Autodesk Inventor part; units mm, degrees
ref_plane "YZ Plane" through (0, 0, 0) normal (1, 0, 0) x (0, 1, 0)
ref_plane "XZ Plane" through (0, 0, 0) normal (0, 1, 0) x (-1, 0, 0)
ref_plane "XY Plane" through (0, 0, 0) normal (0, 0, 1) x (1, 0, 0)
sketch "Szkic1" plane through (0, 0, 0) normal (0, 1, 0) x (-1, 0, 0)
  line L0 (0, 3.2611) -> (1.85, 3.2611)
  line L1 (1.85, 3.2611) -> (2.85, 2.6611)
  line L2 (2.85, 2.6611) -> (2.85, -6.3389)
  line L3 (2.85, -6.3389) -> (6.25, -6.3389)
  line L4 (6.25, -6.3389) -> (6.25, -7.9389)
  line L5 (6.25, -7.9389) -> (3.05, -7.9389)
  line L6 (3.05, -7.9389) -> (3.05, -33.9389)
  line L7 (3.05, -33.9389) -> (2.38, -35.4389)
  line L8 (2.38, -35.4389) -> (2.38, -36.3889)
  line L9 (2.38, -36.3889) -> (0, -38.5259)
  line L10 (0, 3.2611) -> (0, -38.5259)
  point P0 (0, 0)
  dimension "d0" = 1.85
  dimension "d1" = 0.6
  dimension "d2" = 1
  dimension "d3" = 9
  dimension "d4" = 3.4
  dimension "d5" = 1.6
  dimension "d6" = 3.2
  dimension "d7" = 26
  dimension "d8" = 1.5
  dimension "d9" = 0.67
  dimension "d10" = 0.95
  dimension "d11" = 2.137
revolve "Obrót1" add sketch "Szkic1" angle 360 about axis through (0, 0, 3.2611) along (0, 0, -1)
sketch "Szkic2" plane through (0, 0, -6.3389) normal (0, 0, 1) x (1, 0, 0)
  circle A0 centre (0, 0) radius 1.85
  line L0 (5.0074, 2.8738) -> (4.9925, -2.8997)
  line L1 (4.9925, -2.8997) -> (-0.0149, -5.7735)
  line L2 (-0.0149, -5.7735) -> (-5.0074, -2.8738)
  line L3 (-5.0074, -2.8738) -> (-4.9925, 2.8997)
  line L4 (-4.9925, 2.8997) -> (0.0149, 5.7735)
  line L5 (0.0149, 5.7735) -> (5.0074, 2.8738)
  circle A1 centre (0, 0) radius 5
  point P0 (0, 0)
  dimension "d13" = 10
sketch "Szkic3" plane through (0, 0, -7.9389) normal (0, 0, -1) x (-1, 0, 0)
  point P0 (0, 0)
extrude "Wyciągnięcie proste1" add sketch "Szkic2" along normal blind 5.2 contours A0 | L0 L1 A1 | L0 A1 L5 | A1 | A1 L4 L5 | L1 L2 A1 | A1 L3 L4 | L2 L3 A1
thread "Gwint1"
sketch "Szkic4" plane through (0, 0, -7.9389) normal (0, 0, -1) x (-1, 0, 0)
  point P0 (0, 0)
sketch "Szkic5" plane through (5.0074, 2.8738, -1.1389) normal (1, -0.0026, 0) x (0, 0, -1)
  point P0 (-1.1389, -2.8868)
sketch "Szkic6" plane through (0, 0, -7.9389) normal (0, 0, -1) x (-1, 0, 0)
  point P0 (0, 0)
sketch "Szkic7" plane through (5.0074, 2.8738, -1.1389) normal (1, -0.0026, 0) x (0, 0, -1)
  point P0 (-1.1389, -2.8868)
properties part number "śróbki1" material "Stal nierdzewna"
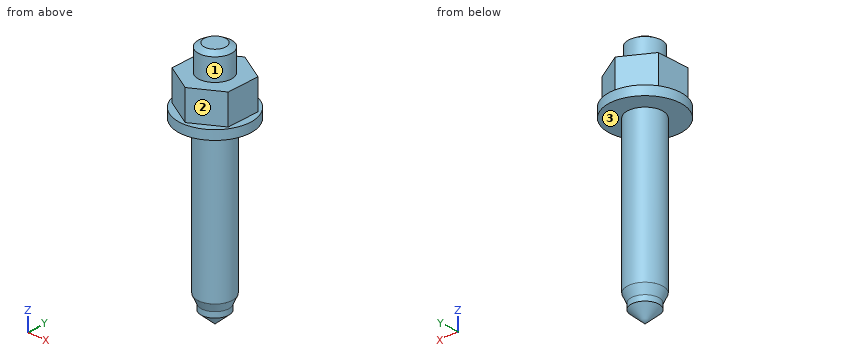
Source: CAD feature listing. Evaluate the final solid. Frame: model axes, mm. Face numbers are marked on the shaded views. A direction names the side the tool comes from. Give positions to 0.01 mm unless a question says otherwise; leave off trailing zeros. Order: outer loops, then holes, each group sorted by start corner. A loop starts at its lowest first (then second) coordinate and runs counter-clockwise, first axis right, second up.
(1) Section query B-B (z = -32.5). Return the cut outline in (x, y).
(2) Section query D-D (z = -4). Return the cut outline in (x, y).
(3) Section query A-A (x = 4.5). Return the cut outline in (y, z), plus the area to 3 significant figures.
(4) Material intervals for line 1 along Z through (x, y) = (2, -5); line 2 along X through (y, z) = (1.25, -1.5); line 3 along Z through (x, y) = (2, 2.5), sorted ascending.
(5) Access query for the marked faces 1, 2 and 3. Directions: +Z, -Z, +X, -X, +Y, -Y. A direction counts if a zero-diameter tool reaches every point of the face in a straight line with its end or side. Return the directions, or none.
(6) Section query C-C (x = -4). Return the cut outline in (y, z).
(7) Contact query for flat-ended pins moving along their axis: P1, Ø1.5, axis at y = -0.5, z = -16.5, coming from the -X side; P2, Ø1, axis at x = 4.5, y = -3.5, coming from the +Z side; P3, Ø1.5, axis at x = -1, z = -13.5, coming from the -Y side. Output: stop coordinate, or through.
Outcome:
1. outline: circle Ø6.1 at (0, 0)
2. outline: (-5.01, -2.87) - (-0.01, -5.77) - (4.99, -2.9) - (5.01, 2.87) - (0.01, 5.77) - (-4.99, 2.9) - close
3. outline: (-4.34, -7.94) - (4.34, -7.94) - (4.34, -6.34) - (3.17, -6.34) - (3.17, -1.14) - (-3.18, -1.14) - (-3.18, -6.34) - (-4.34, -6.34) - close
3. area: 46.9 mm2
4. line 1: z = -7.94 to -6.34
4. line 2: x = -5 to 5
4. line 3: z = -7.94 to -1.14
5. face 1: +Z
5. face 2: +Z, +X, -Y
5. face 3: -Z
6. outline: (-4.8, -7.94) - (4.8, -7.94) - (4.8, -6.34) - (3.47, -6.34) - (3.47, -1.14) - (-3.46, -1.14) - (-3.46, -6.34) - (-4.8, -6.34) - close
7. P1: stops at x = -3.05
7. P2: stops at z = -1.14
7. P3: stops at y = -3.04
